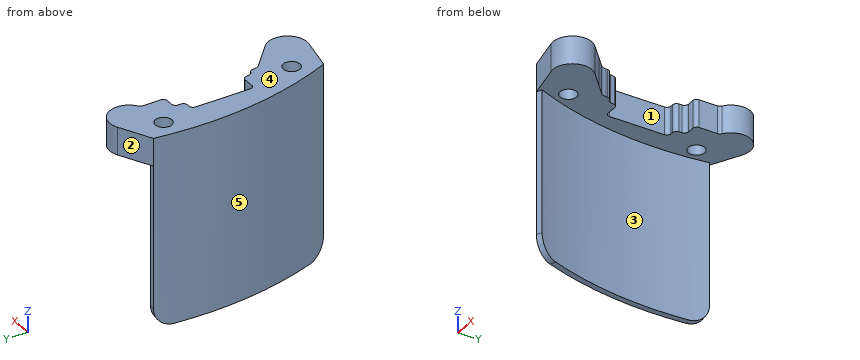
Autodesk Inventor part; units mm, degrees
ref_plane "YZ Plane" through (0, 0, 0) normal (1, 0, 0) x (0, 1, 0)
ref_plane "XZ Plane" through (0, 0, 0) normal (0, 1, 0) x (-1, 0, 0)
ref_plane "XY Plane" through (0, 0, 0) normal (0, 0, 1) x (1, 0, 0)
sketch "Skizze1" plane through (0, 0, 0) normal (0, 0, 1) x (1, 0, 0)
  circle A0 centre (0, 0) radius 88
  circle A1 centre (-82.6842, 7.2339) radius 2.1
  arc A2 (-78.002, 6.8243) -> (-73.5779, -26.7802) centre (0, 0) ccw
  circle A3 centre (-82.6842, 7.2339) radius 4.7
  circle A4 centre (-77.9945, -28.3877) radius 2.1
  circle A5 centre (-77.9945, -28.3877) radius 4.7
  circle A6 centre (0, 0) radius 78.3
  circle A7 centre (0, 0) radius 86.5
  arc A8 (-84.1729, 21.9984) -> (-86.4353, 9.8964) centre (0, 0) ccw
  line L0 (0, 0) -> (-82.0101, 11.8853)
  line L1 (-82.0101, 11.8853) -> (-87.0902, 12.6216)
  line L2 (0, 0) -> (-76.1395, -32.7061)
  line L3 (-76.1395, -32.7061) -> (-80.8559, -34.7321)
  line L4 (0, 0) -> (-82.828, 2.5361)
  line L5 (-82.828, 2.5361) -> (-87.9588, 2.6932)
  line L6 (0, 0) -> (-79.3493, -23.8872)
  line L7 (-79.3493, -23.8872) -> (-84.2646, -25.3669)
  line L8 (-78.3816, 80.7625) -> (-42.1157, 57.6586)
  line L9 (-42.1157, 57.6586) -> (-70.0553, 13.8022)
  line L10 (-70.0553, 13.8022) -> (-106.3212, 36.9061)
  line L11 (-106.3212, 36.9061) -> (-78.3816, 80.7625)
  line L12 (-56.0855, 35.7304) -> (-92.3514, 58.8343) construction
  line L13 (-64.096, -31.4636) -> (-25.7575, -66.5943)
  line L14 (-25.7575, -66.5943) -> (-54.8079, -98.2972)
  line L15 (-54.8079, -98.2972) -> (-93.1463, -63.1665)
  line L16 (-93.1463, -63.1665) -> (-64.096, -31.4636)
  line L17 (-47.7296, -52.0877) -> (-73.9771, -80.7319) construction
  arc A9 (-44.3621, 76) -> (44.3621, 76) centre (0, 0) ccw
  line L18 (13, 63) -> (-13, 63)
  line L19 (0, 63) -> (0, -88)
  line L20 (0, 0) -> (-56.0855, 35.7304) construction
  line L21 (0, 0) -> (-44.9267, -49.0289) construction
  line L22 (0, 0) -> (-88, 0)
  line L23 (0, 0) -> (-86.6631, 15.281) construction
  line L24 (0, 0) -> (-79.7551, -37.1904) construction
  circle A10 centre (0, 0) radius 83 construction
  line L25 (-63.2545, -17.7499) -> (-72.5045, -17.7499)
  arc A11 (-72.5045, -17.7499) -> (-74.5045, -19.7499) centre (-72.5045, -19.7499) ccw
  line L26 (-74.5045, -19.7499) -> (-74.5045, -21.0458)
  arc A12 (-74.5045, -21.0458) -> (-73.8556, -22.5204) centre (-72.5045, -21.0458) ccw
  line L27 (-73.8556, -22.5204) -> (-71.5045, -24.6748)
  line L28 (-71.5045, -24.6748) -> (-52.6253, -41.9744)
  arc A13 (-52.6253, -41.9744) -> (-51.2741, -42.4999) centre (-51.2741, -40.4999) ccw
  line L29 (-51.2741, -42.4999) -> (51.2741, -42.4999)
  arc A14 (51.2741, -42.4999) -> (52.6253, -41.9744) centre (51.2741, -40.4999) ccw
  line L30 (52.6253, -41.9744) -> (71.5045, -24.6748)
  line L31 (71.5045, -24.6748) -> (73.8557, -22.5204)
  arc A15 (73.8557, -22.5204) -> (74.5045, -21.0458) centre (72.5045, -21.0458) ccw
  line L32 (74.5045, -21.0458) -> (74.5045, -19.7499)
  arc A16 (74.5045, -19.7499) -> (72.5045, -17.7499) centre (72.5045, -19.7499) ccw
  line L33 (72.5045, -17.7499) -> (63.2545, -17.7499)
  arc A17 (61.2545, -15.7499) -> (63.2545, -17.7499) centre (63.2545, -15.7499) ccw
  line L34 (61.2545, -15.7499) -> (61.2545, -2.2499)
  arc A18 (63.2545, -0.2499) -> (61.2545, -2.2499) centre (63.2545, -2.2499) ccw
  line L35 (63.2545, -0.2499) -> (72.5045, -0.2499)
  arc A19 (72.5045, -0.2499) -> (74.5045, 1.7501) centre (72.5045, 1.7501) ccw
  line L36 (74.5045, 1.7501) -> (74.5045, 6.2357)
  arc A20 (74.5045, 6.2357) -> (74.1913, 7.3103) centre (72.5045, 6.2357) ccw
  line L37 (74.1913, 7.3103) -> (66.8685, 18.8046)
  line L38 (66.8685, 18.8046) -> (66.8312, 18.8625)
  line L39 (66.8312, 18.8625) -> (63.3633, 24.3061)
  line L40 (63.3633, 24.3061) -> (61.5013, 27.2292)
  arc A21 (61.5013, 27.2292) -> (61.4647, 27.2866) centre (58.5872, 25.413) ccw
  line L41 (61.4647, 27.2866) -> (59.6025, 30.21)
  line L42 (59.6025, 30.21) -> (59.5849, 30.2372)
  line L43 (59.5849, 30.2372) -> (52.3622, 41.5747)
  arc A22 (52.3622, 41.5747) -> (50.6754, 42.5001) centre (50.6754, 40.5001) ccw
  line L44 (50.6754, 42.5001) -> (34.4476, 42.5001)
  arc A23 (33.1728, 42.9591) -> (34.4476, 42.5001) centre (34.4477, 44.5002) ccw
  arc A24 (33.1728, 42.9591) -> (28.0733, 42.9591) centre (30.623, 39.877) ccw
  arc A25 (26.7984, 42.5001) -> (28.0733, 42.9591) centre (26.7984, 44.5002) ccw
  line L45 (26.7984, 42.5001) -> (-26.7984, 42.5001)
  arc A26 (-28.0733, 42.9591) -> (-26.7984, 42.5001) centre (-26.7984, 44.5002) ccw
  arc A27 (-28.0733, 42.9591) -> (-33.1728, 42.9591) centre (-30.623, 39.877) ccw
  arc A28 (-34.4476, 42.5001) -> (-33.1728, 42.9591) centre (-34.4477, 44.5002) ccw
  line L46 (-34.4476, 42.5001) -> (-50.6754, 42.5001)
  arc A29 (-50.6754, 42.5001) -> (-52.3622, 41.5747) centre (-50.6754, 40.5001) ccw
  line L47 (-52.3622, 41.5747) -> (-59.5849, 30.2372)
  line L48 (-59.5849, 30.2372) -> (-59.6025, 30.21)
  line L49 (-59.6025, 30.21) -> (-61.4647, 27.2866)
  arc A30 (-61.4647, 27.2866) -> (-61.5013, 27.2292) centre (-58.5191, 25.37) ccw
  line L50 (-61.5013, 27.2292) -> (-63.3633, 24.3061)
  line L51 (-63.3633, 24.3061) -> (-66.8312, 18.8625)
  line L52 (-66.8312, 18.8625) -> (-66.8685, 18.8046)
  line L53 (-66.8685, 18.8046) -> (-74.1912, 7.3103)
  arc A31 (-74.1912, 7.3103) -> (-74.5045, 6.2357) centre (-72.5045, 6.2357) ccw
  line L54 (-74.5045, 6.2357) -> (-74.5045, 1.7501)
  arc A32 (-74.5045, 1.7501) -> (-72.5045, -0.2499) centre (-72.5045, 1.7501) ccw
  line L55 (-72.5045, -0.2499) -> (-63.2545, -0.2499)
  arc A33 (-61.2545, -2.2499) -> (-63.2545, -0.2499) centre (-63.2545, -2.2499) ccw
  line L56 (-61.2545, -2.2499) -> (-61.2545, -15.7499)
  arc A34 (-63.2545, -17.7499) -> (-61.2545, -15.7499) centre (-63.2545, -15.7499) ccw
  line L57 (-82.6842, 7.2339) -> (-80.4481, 20.4232)
  circle A35 centre (-76.8409, 12.298) radius 4.9146
  circle A36 centre (-76.8409, 12.298) radius 4
  line L58 (-74.5045, 1.7501) -> (-78.2804, 1.7501)
  line L59 (-74.5045, -19.7499) -> (-75.7683, -19.7499)
  line L60 (-87.0902, 12.6216) -> (-79.059, 16.6835)
  line L61 (-77.9945, -28.3877) -> (-72.421, -40.5488)
  circle A37 centre (-71.0396, -31.7667) radius 4.9146
  circle A38 centre (-71.0396, -31.7667) radius 4
  line L62 (-80.8559, -34.7321) -> (-72.0471, -36.577)
  line L63 (-74.5045, 6.2357) -> (-74.5045, 10.7976)
  line L64 (-77.9945, -28.3877) -> (-73.2945, -28.3877)
  line L65 (-73.2945, -28.3877) -> (-73.2945, -31.484)
  line L66 (-73.2945, -28.3877) -> (-73.2945, -23.0346)
  point P0 (0, 0)
  point P1 (-85.6057, 12.4064)
  point P2 (-79.4777, -34.1401)
  point P3 (0, 0)
  point P4 (-74.9054, -43.26)
  point P5 (-83.5496, 22.399)
  point P6 (-86.1005, 12.4781)
  point P7 (-86.4122, 10.096)
  point P8 (-71.9434, -30.9037)
  point P9 (-77.4904, 11.2303)
  point P10 (-72.696, 9.6574)
  point P11 (-67.7194, -28.1432)
  point P12 (-67.103, -28.8245)
  point P13 (-74.5045, 7.9743)
  dimension "d0" = 9.4
  dimension "d1" = 173
  dimension "d8" = 52
  dimension "d9" = 43
  dimension "d10" = 43
  dimension "d11" = 52
  dimension "d12" = 66.5
  dimension "d13" = 90
  dimension "d14" = 90
  dimension "d15" = 90
  dimension "d16" = 90
  dimension "d17" = 90
  dimension "d18" = 90
  dimension "d19" = 90
  dimension "d20" = 66.5
  dimension "d21" = 26
  dimension "d22" = 47.5
  dimension "d23" = 32.5
  dimension "d139" = 10
  dimension "d140" = 25
  dimension "d156" = 8
  dimension "d157" = 8
extrude "Extrusion1" add sketch "Skizze1" against normal blind 41 contours A0 L7 A7 A5 L3 | L1 A8 A3 A7 L5 A0 | A0 L22 A7 L7 | L5 A7 L22 A0 | L1 A7 A3 A8 | A5 A7 | A3 A7
extrude "Extrusion2" add sketch "Skizze1" along normal blind 7 contours A0 L7 A7 A5 L3 | L3 A7 L62 | L1 A8 A3 A7 L5 A0 | L60 A8 L1 | A0 L22 A7 L7 | L3 A5 L61 L62 A7 | A7 A5 L3 | L5 A7 L22 A0 | L1 A7 A3 A8 | A8 L60 A7 L1 | L60 L57 A3 L1 A7 | L7 A5 A7 | A7 L22 A2 L6 L7 | A7 A5 A37 L64 A4 L61 | A5 A7 | L61 A37 L62 | A37 L2 A38 A6 | A6 A38 L2 A37 | L54 L58 A2 L4 | L4 A2 A6 A35 L63 L54 | A12 L27 L66 A37 A6 A2 L6 | L6 A2 L59 L26 A12 | L5 L4 A2 L22 A7 | A7 A3 L5 | A3 A7 | L1 A3 A7 | L60 A35 L57 | A35 L0 A36 A6 | A6 A36 L0 A35 | L6 A2 A5 | L61 A4 L64 A37 A5 | A5 A37 L2 | L2 A37 L61 | A38 L2 A6 | A6 L2 A38 | A35 L63 A36 L0 | L2 A38 A6 L66 A37 | A37 L66 L27 L28 | L4 A3 A2 | A7 A3 A35 | A35 L0 L57 | A36 L0 A6 | A6 L0 A36 | A6 A37 A5 | A37 L64 A5 A38 | A5 A38 L2 A37 | L2 L65 A38 A6 | A6 A38 L2 | A38 A5 L65 L2 | A36 L63 L0 | A35 A6 A36 L63 | L66 A6 A37 | A3 A35 A6 | L0 A35 A3 | L0 A36 A3 A35 | L0 L63 A36 A6 | A6 A36 A3 L0 | A37 A6 L66 A5 | A5 L64 A37 | A38 A5 | A38 A5 L66 A6 | A35 A3 A36 A6 | A3 A36 A35 | A3 A36
sketch "Skizze7" plane through (0, 0, 7) normal (0, 0, 1) x (1, 0, 0)
  arc A0 (-75.2406, -20.5635) -> (-69.3003, -22.9246) centre (-71.3821, -19.509) ccw
  arc A1 (-77.999, 0.3892) -> (-75.2406, -20.5635) centre (0, 0) ccw
  arc A2 (-72.8723, 4.2072) -> (-77.999, 0.3892) centre (-73.9991, 0.3692) ccw
  arc A3 (-72.8723, 4.2072) -> (-61.6214, 8.4293) centre (-70.0553, 13.8022) ccw
  arc A4 (-73.0131, 3.7275) -> (-61.1997, 8.1606) centre (-70.0553, 13.8022) ccw
  arc A5 (-73.0131, 3.7275) -> (-77.499, 0.3867) centre (-73.9991, 0.3692) ccw
  arc A6 (-77.499, 0.3867) -> (-74.7582, -20.4317) centre (0, 0) ccw
  arc A7 (-74.7582, -20.4317) -> (-69.5605, -22.4976) centre (-71.3821, -19.509) ccw
  arc A8 (-57.0023, -23.7222) -> (-69.5605, -22.4976) centre (-64.096, -31.4636) ccw
  line L0 (-81.0045, -17) -> (-62.0045, -17)
  line L1 (-62.0045, -17) -> (-62.0045, -1)
  line L2 (-62.0045, -1) -> (-81.0045, -1)
  line L3 (-81.0045, -1) -> (-81.0045, -17)
  line L4 (-81.0045, -17) -> (-62.0045, -1) construction
  line L5 (-62.0045, -17) -> (-81.0045, -1) construction
  arc A9 (-75.2406, -20.5635) -> (-69.3003, -22.9246) centre (-71.3821, -19.509) ccw
  arc A10 (-77.999, 0.3892) -> (-75.2406, -20.5635) centre (0, 0) ccw
  arc A11 (-72.8723, 4.2072) -> (-77.999, 0.3892) centre (-73.9991, 0.3692) ccw
  arc A12 (-72.8723, 4.2072) -> (-61.6214, 8.4293) centre (-70.0553, 13.8022) ccw
  arc A13 (-73.0131, 3.7275) -> (-61.1997, 8.1606) centre (-70.0553, 13.8022) ccw
  arc A14 (-73.0131, 3.7275) -> (-77.499, 0.3867) centre (-73.9991, 0.3692) ccw
  arc A15 (-77.499, 0.3867) -> (-74.7582, -20.4317) centre (0, 0) ccw
  arc A16 (-74.7582, -20.4317) -> (-69.5605, -22.4976) centre (-71.3821, -19.509) ccw
  arc A17 (-57.0023, -23.7222) -> (-69.5605, -22.4976) centre (-64.096, -31.4636) ccw
  line L6 (0, 0) -> (-88, 0) construction
  line L7 (0, 0) -> (-70.4769, -25.6515) construction
  line L8 (0, 0) -> (-74.7146, 6.5367) construction
  circle A18 centre (-74.7146, 6.5367) radius 3
  line L9 (-74.7146, 6.5367) -> (-74.7146, -9.8771) construction
  line L10 (-78.7146, 6.5367) -> (-78.7146, -9.8771)
  line L11 (-70.7146, -9.8771) -> (-70.7146, 6.5367)
  arc A19 (-78.7146, -9.8771) -> (-70.7146, -9.8771) centre (-74.7146, -9.8771) ccw
  line L12 (-70.4769, -25.6515) -> (-70.4769, -13.0481) construction
  line L13 (-66.4769, -25.6515) -> (-66.4769, -13.0481)
  line L14 (-74.4769, -13.0481) -> (-74.4769, -25.6515)
  arc A20 (-66.4769, -13.0481) -> (-74.4769, -13.0481) centre (-70.4769, -13.0481) ccw
  point P0 (83.6944, 461.4718)
  point P1 (50.4138, 461.4718)
  point P2 (51.6944, 461.4718)
  point P3 (82.4138, 461.4718)
  point P4 (225.0044, 602.8331)
  point P5 (191.7237, 602.8331)
  point P6 (193.0044, 602.8331)
  point P7 (223.7237, 602.8331)
  point P8 (363.5869, 628.2091)
  point P9 (357.6097, 628.732)
  point P10 (362.0169, 595.2563)
  point P11 (367.655, 597.3084)
  point P12 (406.3129, 669.9339)
  point P13 (410.3051, 673.6839)
  point P14 (281.6601, 684.5107)
  point P15 (276.0219, 682.4586)
  point P16 (276.7768, 680.2764)
  point P17 (229.3797, 602.3331)
  point P18 (240.8641, 609.8331)
  point P19 (280.2544, 653.8611)
  point P20 (280.0901, 651.5579)
  point P21 (286.0672, 651.035)
  point P22 (286.3631, 657.444)
  point P23 (283.6046, 678.3966)
  point P24 (208.3641, 735.8331)
  point P25 (208.3641, 713.8331)
  point P26 (208.3641, 669.8331)
  point P27 (208.3641, 666.8331)
  point P28 (208.3641, 602.3331)
  point P29 (-74.7146, -1.6702)
  point P30 (-70.4769, -19.3498)
  point P31 (-61.892, 765.0568)
  point P32 (-53.892, 765.0568)
  point P33 (-66.1297, 787.0568)
  point P34 (-58.1297, 787.0568)
  point P35 (280.1559, 614.5868)
  point P36 (280.8975, 610.8357)
  point P37 (282.7456, 598.5868)
  dimension "d88" = 19
  dimension "d89" = 16
  dimension "d106" = 8
  dimension "d107" = 8
extrude "Extrusion6" cut sketch "Skizze7" against normal blind 41 contours L0 L3 L2 L10 A19 A1 | A1 A19 A6 L0 | A19 L10 L2 A1 | A1 L2 A6 A19 | A6 A19 L14 L0 | L14 A19 L11 A20 L13 L0 | A6 L2 L11 A20 L14 A19 | L13 A20 L11 L2 L1 L0 | L14 A20 L11 A19
fillet "Rundung2" radius 1 9 edges at (-81.0045, -17, 3.5) (-81.0045, -1, 3.5) (-78.2936, -1, 3.5) (-78.2804, 1.7501, 3.5) (-74.5045, 1.7501, 3.5) (-76.4323, -17, 3.5) (-75.7683, -19.7499, 3.5) (-74.5045, -19.7499, 3.5) (-74.5045, 7.9743, 3.5)
fillet "Rundung3" radius 5 2 edges at (-86.3479, 12.514, -41) (-80.1668, -34.4361, -41)
equation "\"d10\" = d9"
equation "\"d11\" = d8"
properties part number "Abdeckung"
Input: part model. Units: mm. Frame: model coordinates. Face numbers are marked on the shaded views. A direction names the side the tool comes from. Give positions to 0.01 mm unless a question says otherwise; leave off trailing zeros. Write each loop counter-clockwise with the first axis right and the second up, starting at its lowest first coordinate (ties: lowest second). Pieces come first, ordered by that corner, then holes. Notation, with made-up numbers: M 78,29.5 L 86,29.5 A13 cw 86,41.5 Z; hole C 9.25,77.25 d6. An arc over 180 degrees is marked long. Use one line per item in the form item = value.
1. Cut plane B-B on z = 4.5. State how many separate pieces and enclosed holes the cut face has, and give its area (3 significant figures).
Outcome:
separate_pieces = 1
enclosed_holes = 2
area = 549 mm²
2. Cut plane D-D on z = -33. Return loops of the section in (x, y), and give its area (3 significant figures).
Outcome:
outline = M -87.09,12.62 A88 ccw -80.86,-34.73 L -79.48,-34.14 A86.5 cw -85.61,12.41 Z
area = 71.9 mm²
3. Cut plane A-A on y = -12.5. Return loops of the section in (x, z).
Outcome:
outline = M -87.11,-41 L -85.59,-41 L -85.59,0 L -81,0 L -81,7 L -87.11,7 Z
4. Cut plane C-C on x = -68.75. Return loops of the section in (y, z).
Outcome:
outline = M -36.12,0 L -27.2,0 L -27.2,7 L -36.12,7 Z
5. Mould query, pull axis Y, two halves, no side actions, for the marked faces 3, 4 and 5. Classes: released by +Y, released by -Y, zero draft, split by the parting line, or undercut.
Outcome:
face_3 = undercut
face_4 = zero draft
face_5 = split by the parting line
6. Ray query, L1, parallel to Z at x = -79.25, y = 7; L2, parallel to X at y = 2, z = -37.5; L3, parallel to X at y = -23, z = 3.5. Return the intervals inside material, ascending.
Outcome:
L1 = 0 to 7
L2 = -87.98 to -86.48
L3 = -84.94 to -73.33
7. Reachability of the marked faces 1 and 2 from +Z, -Z, +X, -X, +Y, -Y: full face, straight path, thin tool, end or side. Return the list, or none.
Outcome:
face_1 = +Z, -Z, +X
face_2 = +Z, -Z, -X, +Y
8. First-contact query: P1, Ø2.5, axis at y = 4.5, z = 4.5, coming from the +X side; P2, Ø6, axis at x = -80.5, z = -8.5, coming from the -Y side; P3, Ø0.5, axis at x = -76.5, z = 4, coming from the -Y side; P4, Ø1.5, axis at x = -77.5, z = -23, coming from the -Y side. Flat tips, straight axial feed; report the tip coordinate or a pass-through.
Outcome:
P1 = -74.5
P2 = -34.73
P3 = -35.7
P4 = through
